```python
from build123d import *

# Parameters (mm, degrees)
F0_W         = 279.4
F0_H         = 482.6
F1_DEPTH     = 381
F2_T         = -7.62
F3_W         = 264.16
F3_H         = 30.1203280687
F4_DEPTH     = 355.6
F5_W         = 102.4026331621
F5_H         = 105.4210998118
F6_DEPTH     = 177.8
F7_DEPTH     = 177.8
F8_T         = 7.62
F8_T3_DEPTH  = 388.62
F8_T5_DEPTH  = 42.9501895142
F8_T7_DEPTH  = 370.84
F8_T9_DEPTH  = 45.3603280687
F8_T11_DEPTH = 146.3519571328
F8_T13_DEPTH = 193.04
F8_T15_DEPTH = 188.2364254725
F8_T17_DEPTH = 279.4
F8_T19_DEPTH = 424.7694824171
F8_T21_DEPTH = 117.6426331621
F8_T23_DEPTH = 120.6610998118


# Not quite as in the source:
# - a shell that OpenCascade refuses in one call is made with other operations: the cavity is built on its own and cut out


with BuildPart() as f1:
    # F0 (on Front) → F1 (new body)
    with BuildSketch(Plane.XZ):
        Rectangle(F0_W, F0_H)
    extrude(amount=F1_DEPTH)

    # F2
    f2_openings = [f1.faces().sort_by_distance(p)[0] for p in [
        (0, -381, 0),
    ]]
    offset(amount=F2_T, openings=f2_openings)

    # F3 (on face) → F4 (join)
    with BuildSketch(Plane.XZ.offset(7.62)):
        with Locations((0, -190.9096464515)):
            Rectangle(F3_W, F3_H)
    extrude(amount=F4_DEPTH)

    # F5 (on face) → F6 (join)
    with BuildSketch(Plane.XZ.offset(7.62)):
        with Locations((80.8786834189, 7.9730246216)):
            Rectangle(F5_W, F5_H)
    extrude(amount=F6_DEPTH)

    # F7 (add): a face of the model
    f7_faces = [f1.faces().sort_by_distance(p)[0] for p in [
        (80.8786834189, -185.42, 7.9730246216),
    ]]
    extrude(f7_faces, amount=-F7_DEPTH)

    # F8: shell of thickness 7.62, made by hand


with BuildPart() as f8_core1:
    # F8_t2: copy of F1
    add(f1.part)

    # the walls: a layer under each face that stays
    f8_faces = [f8_core1.faces().sort_by_distance(p)[0] for p in [
        (139.7, -190.5, 0),
        (0, -190.5, -241.3),
        (0, -190.5, 241.3),
        (0, 0, 0),
        (96.04375, -381, -235.3419753086),
        (-139.7, -190.5, 0),
        (132.08, -194.31, 0),
        (0, -194.31, -233.68),
        (-132.08, -194.31, 0),
        (0, -194.31, 233.68),
        (0, -7.62, -219.8249052429),
        (0, -185.42, -205.9698104858),
        (0, -363.22, -190.9096464515),
        (0, -185.42, -175.8494824171),
        (0, -7.62, 28.9152587914),
        (80.8786834189, -96.52, -44.7375252843),
        (80.8786834189, -96.52, 60.6835745275),
        (29.6773668379, -96.52, 7.9730246216),
    ]]
    thicken(f8_faces, amount=-F8_T, mode=Mode.SUBTRACT)

    # F8_s4 → F8_t3 (cut)
    with BuildSketch(Plane.XZ):
        Polygon((132.0038, -233.6038), (139.7, -233.68), (139.7, -241.3), (132.08, -241.3), align=None)
        Polygon((132.0038, 233.6038), (139.7, 233.68), (139.7, 241.3), (132.08, 241.3), align=None)
        Polygon((-132.0038, -233.6038), (-132.08, -241.3), (-139.7, -241.3), (-139.7, -233.68), align=None)
        Polygon((-132.0038, 233.6038), (-139.7, 233.68), (-139.7, 241.3), (-132.08, 241.3), align=None)
    extrude(amount=F8_T3_DEPTH, mode=Mode.SUBTRACT)

    # F8_s6 → F8_t5 (cut)
    with BuildSketch(Plane.XY.offset(-241.3)):
        Polygon((132.0038, -7.6962), (139.7, -7.62), (139.7, 0), (132.08, 0), align=None)
        Polygon((-132.0038, -7.6962), (-139.7, -7.62), (-139.7, 0), (-132.08, 0), align=None)
    extrude(amount=F8_T5_DEPTH, mode=Mode.SUBTRACT)

    # F8_s8 → F8_t7 (cut)
    with BuildSketch(Plane.XZ):
        Polygon((132.0038, -206.0460104858), (139.7, -205.9698104858), (139.7, -198.3498104858), (132.08, -198.3498104858), align=None)
        Polygon((132.0038, -175.7732824171), (139.7, -175.8494824171), (139.7, -183.4694824171), (132.08, -183.4694824171), align=None)
        Polygon((-132.0038, -175.7732824171), (-139.7, -175.8494824171), (-139.7, -183.4694824171), (-132.08, -183.4694824171), align=None)
        Polygon((-132.0038, -206.0460104858), (-139.7, -205.9698104858), (-139.7, -198.3498104858), (-132.08, -198.3498104858), align=None)
    extrude(amount=F8_T7_DEPTH, mode=Mode.SUBTRACT)

    # F8_s10 → F8_t9 (cut)
    with BuildSketch(Plane.XY.offset(-213.5898104858)):
        Polygon((132.0038, -363.2962), (139.7, -363.22), (139.7, -355.6), (132.08, -355.6), align=None)
        Polygon((-132.0038, -363.2962), (-139.7, -363.22), (-139.7, -355.6), (-132.08, -355.6), align=None)
    extrude(amount=F8_T9_DEPTH, mode=Mode.SUBTRACT)

    # F8_s12 → F8_t11 (cut)
    with BuildSketch(Plane.XY.offset(-183.4694824171)):
        Polygon((132.0038, -7.6962), (139.7, -7.62), (139.7, 0), (132.08, 0), align=None)
    extrude(amount=F8_T11_DEPTH, mode=Mode.SUBTRACT)

    # F8_s14 → F8_t13 (cut)
    with BuildSketch(Plane.XZ):
        Polygon((132.0038, -44.8137252843), (139.7, -44.7375252843), (139.7, -37.1175252843), (132.08, -37.1175252843), align=None)
        Polygon((132.0038, 60.7597745275), (139.7, 60.6835745275), (139.7, 53.0635745275), (132.08, 53.0635745275), align=None)
    extrude(amount=F8_T13_DEPTH, mode=Mode.SUBTRACT)

    # F8_s16 → F8_t15 (cut)
    with BuildSketch(Plane.XY.offset(53.0635745275)):
        Polygon((132.0038, -7.6962), (139.7, -7.62), (139.7, 0), (132.08, 0), align=None)
    extrude(amount=F8_T15_DEPTH, mode=Mode.SUBTRACT)

    # F8_s18 → F8_t17 (cut)
    with BuildSketch(Plane.YZ.offset(-139.7)):
        Polygon((-7.6962, -233.6038), (-7.62, -241.3), (0, -241.3), (0, -233.68), align=None)
        Polygon((-7.6962, 233.6038), (-7.62, 241.3), (0, 241.3), (0, 233.68), align=None)
        Polygon((-7.6962, -206.0460104858), (0, -205.9698104858), (0, -198.3498104858), (-7.62, -198.3498104858), align=None)
        Polygon((-7.6962, -175.7732824171), (-7.62, -183.4694824171), (0, -183.4694824171), (0, -175.8494824171), align=None)
    extrude(amount=F8_T17_DEPTH, mode=Mode.SUBTRACT)

    # F8_s20 → F8_t19 (cut)
    with BuildSketch(Plane.XY.offset(-183.4694824171)):
        Polygon((-132.0038, -7.6962), (-139.7, -7.62), (-139.7, 0), (-132.08, 0), align=None)
    extrude(amount=F8_T19_DEPTH, mode=Mode.SUBTRACT)

    # F8_s22 → F8_t21 (cut)
    with BuildSketch(Plane.YZ.offset(22.0573668379)):
        Polygon((-7.6962, 60.7597745275), (0, 60.6835745275), (0, 53.0635745275), (-7.62, 53.0635745275), align=None)
        Polygon((-7.6962, -44.8137252843), (0, -44.7375252843), (0, -37.1175252843), (-7.62, -37.1175252843), align=None)
    extrude(amount=F8_T21_DEPTH, mode=Mode.SUBTRACT)

    # F8_s24 → F8_t23 (cut)
    with BuildSketch(Plane.XY.offset(-52.3575252843)):
        Polygon((29.6011668379, -7.6962), (29.6773668379, 0), (37.2973668379, 0), (37.2973668379, -7.62), align=None)
    extrude(amount=F8_T23_DEPTH, mode=Mode.SUBTRACT)


with BuildPart() as f1_1:
    add(f1.part)

    # what is left inside the walls is the cavity
    f8_cavity = [f8_core1.part.solids().sort_by_distance(p)[0] for p in [
        (84.688683, -126.153333, 52.987375),
        (0, -239.606667, -183.545682),
    ]]
    add(f8_cavity, mode=Mode.SUBTRACT)


solid = f1_1.part
```
Geometry check sheet. Reference: the model listing, model coordinates, mm. A direction names the side the tool comes from. Coordinates: 2 decimals unless noted, no trailing zeros. Order: outer loops, then holes, each group sorted by start corner. A loop starts at its lowest first (then second) coordinate and runs counter-clockwise, first axis right, second up. Notation, with made-up numbers: M 32,-23.5 L 48,-23.5 A12 ccw 48,-11.5 Z; hole C -28.5,18.25 d4. An arc over 180 degrees is marked long. Answer as a JSON object with one key per item and string values.
Q1. Cross-section at C-C on z = 173. Record the cut outline in (x, y).
Results are:
{"outline": "M -139.7,-381 L -132.08,-381 L -132.08,-7.62 L 132.08,-7.62 L 132.08,-381 L 139.7,-381 L 139.7,0 L -139.7,0 Z"}
Q2. Cross-section at A-A on x = 65.5. Record the cut outline in (y, z).
Results are:
{"outline": "M -381,-241.3 L 0,-241.3 L 0,241.3 L -381,241.3 L -381,233.68 L -7.62,233.68 L -7.62,60.68 L -185.42,60.68 L -185.42,53.06 L -7.62,53.06 L -7.62,-37.12 L -185.42,-37.12 L -185.42,-44.74 L -7.62,-44.74 L -7.62,-175.85 L -363.22,-175.85 L -363.22,-205.97 L -7.62,-205.97 L -7.62,-233.68 L -381,-233.68 Z; hole M -355.6,-198.35 L -7.62,-198.35 L -7.62,-183.47 L -355.6,-183.47 Z"}
Q3. Tool access check on faces 4 (the flat face through (84, -95, 53.064)), 5 (the flat face through (-132.08, -179, -191)), 6 (the flat face through (-2, -188, -241.3)). Record the directions out of +Z, -Z, +X, -X, +Y, -Y that give a thin tool (end or side, any length) a straight path to the whole face; none if there is none.
Results are:
{"face 4": "-Y", "face 5": "none", "face 6": "-Z, +X, -X, +Y, -Y"}
Q4. Cross-section at B-B on y = -140.5. Record the cut outline in (x, z), and give its area (3 significant figures).
Results are:
{"outline": "M -139.7,-241.3 L 139.7,-241.3 L 139.7,241.3 L -139.7,241.3 Z; hole M -132.08,-233.68 L 132.08,-233.68 L 132.08,-205.97 L -132.08,-205.97 Z; hole M -132.08,-198.35 L 132.08,-198.35 L 132.08,-183.47 L -132.08,-183.47 Z; hole M -132.08,-175.85 L 132.08,-175.85 L 132.08,-44.74 L 29.68,-44.74 L 29.68,60.68 L 132.08,60.68 L 132.08,233.68 L -132.08,233.68 Z; hole M 37.3,-37.12 L 132.08,-37.12 L 132.08,53.06 L 37.3,53.06 Z", "area": "17,700 mm²"}
Q5. Cross-section at D-D on y = -246.5. Record the cut outline in (x, z), and give its area (3 significant figures).
Results are:
{"outline": "M -139.7,-241.3 L 139.7,-241.3 L 139.7,241.3 L -139.7,241.3 Z; hole M -132.08,-233.68 L 132.08,-233.68 L 132.08,-205.97 L -132.08,-205.97 Z; hole M -132.08,-198.35 L 132.08,-198.35 L 132.08,-183.47 L -132.08,-183.47 Z; hole M -132.08,-175.85 L 132.08,-175.85 L 132.08,233.68 L -132.08,233.68 Z", "area": "15,400 mm²"}
Q6. Scan lines: line 1 (Z direction, x = 73.5, y = -306.5); line 2 (Z direction, x = 46, y = -42.5); line 3 (X direction, y = -179, z = -106). Record each from-to range of solid material in increasing order.
Results are:
{"line 1": "z = -241.3 to -233.68, -205.97 to -198.35, -183.47 to -175.85, 233.68 to 241.3", "line 2": "z = -241.3 to -233.68, -205.97 to -198.35, -183.47 to -175.85, -44.74 to -37.12, 53.06 to 60.68, 233.68 to 241.3", "line 3": "x = -139.7 to -132.08, 132.08 to 139.7"}
Q7. Release check for a two-part mould opening along Y. For faces 1 (the flat face through (132.08, -179, -191)), 2 (the flat face through (-2, -7.62, -220)), 3 (the flat face through (80, -95, 60.684)) record: released by +Y, released by -Y, zero draft, split by the parting line, or undercut.
Results are:
{"face 1": "undercut", "face 2": "released by -Y", "face 3": "zero draft"}
